For this review, take the finished solid that the model builds, in its own axes (mm). Round coordinates to 2 decimals unless told otherwise and drop trailing zeros. Write each loop counter-clockwise with the first axis right and the second up, starting at its lowest first coordinate (ties: lowest second). Pieces come first, ordered by that corner, then holes. Notation, with made-up numbers: M 36,78.25 L 92,78.25 A19 ccw 92,112.25 Z; hole C 47.25,-12 d1. An arc over 180 degrees is marked long. Use one line per item in the form item = value. Start each with the question number.
Item 1: Add section D-D (x = -52). State the section outline as (y, z) points, and give its area (3 significant figures).
Item 2: Add section A-A (z = -0.65). State the section outline as (x, y) points, and give its area (3 significant figures).
Item 3: Add section B-B (y = 0). State the section outline as (x, z) points.
Item 4: For line 1 (Y direction, x = -47, z = -0.8); line 2 (Y direction, x = -19, z = -0.4); line 3 (Y direction, x = -24, z = -0.65), list the stretches that pass through material, from the lowest coordinate up. Write a range as [from, to].
Item 5: Add section C-C (y = 40). State the section outline as (x, z) points, and give its area (4 significant figures).
Item 6: Draft analysis for pull direction X (two halves, no side actions). For faces 1 (the cylindrical face through (39.54, 40.11, -0.49)), 2 (the cylindrical face through (51.464, -48.985, -0.493)), 3 (the cylindrical face through (-21.66, 0.11, -0.49)), 4 (the flat face through (20, 4, 0)), state which applies: released by +X, released by -X, zero draft, split by the parting line, or undercut.
from build123d import *

# Parameters (mm, degrees)
SKETCH2_R          = 2.5
SKETCH2_R_2        = 2.25
BASE_FLANGE1_DEPTH = 1


# Sheet-metal steps are written as plain solids
with BuildPart() as part:
    # Sketch2 → Base-Flange1 (new body)
    with BuildSketch(Plane.XY):
        with BuildLine():
            Line((-62.163787728, 10), (13.698785388, 10))
            ThreePointArc((13.698785388, 10), (16.546759576, 10.890371912), (18.380431275, 13.244382792))
            Line((18.380431275, 13.244382792), (30.947144181, 46.755617208))
            ThreePointArc((30.947144181, 46.755617208), (32.78081588, 49.109628088), (35.628790069, 50))
            Line((35.628790069, 50), (48.443634474, 50))
            ThreePointArc((48.443634474, 50), (51.428287122, 49.011464641), (53.2327659, 46.436739428))
            Line((53.2327659, 46.436739428), (66.7327659, 1.436739428))
            ThreePointArc((66.7327659, 1.436739428), (66.943634474, 0), (66.7327659, -1.436739428))
            Line((66.7327659, -1.436739428), (53.2327659, -46.436739428))
            ThreePointArc((53.2327659, -46.436739428), (51.428287122, -49.011464641), (48.443634474, -50))
            Line((48.443634474, -50), (35.628790069, -50))
            ThreePointArc((35.628790069, -50), (32.78081588, -49.109628088), (30.947144181, -46.755617208))
            Line((30.947144181, -46.755617208), (18.380431275, -13.244382792))
            ThreePointArc((18.380431275, -13.244382792), (16.546759576, -10.890371912), (13.698785388, -10))
            Line((13.698785388, -10), (-62.163787728, -10))
            ThreePointArc((-62.163787728, -10), (-65.699321634, -8.535533906), (-67.163787728, -5))
            Line((-67.163787728, -5), (-67.163787728, 5))
            ThreePointArc((-67.163787728, 5), (-65.699321634, 8.535533906), (-62.163787728, 10))
        make_face()
        with Locations((-19.163787728, 0)):
            Circle(SKETCH2_R, mode=Mode.SUBTRACT)
        with Locations((42.036212272, 40)):
            Circle(SKETCH2_R, mode=Mode.SUBTRACT)
        with Locations((42.036212272, -40)):
            Circle(SKETCH2_R, mode=Mode.SUBTRACT)
        with Locations((-62.163787728, 0)):
            Circle(SKETCH2_R_2, mode=Mode.SUBTRACT)
        with Locations((-47.163787728, 0)):
            Circle(SKETCH2_R_2, mode=Mode.SUBTRACT)
        with Locations((8.836212272, 0)):
            Circle(SKETCH2_R_2, mode=Mode.SUBTRACT)
        with Locations((60.836212272, 0)):
            Circle(SKETCH2_R_2, mode=Mode.SUBTRACT)
    extrude(amount=-BASE_FLANGE1_DEPTH)


solid = part.part
Calculated:
q1.outline = M -10,-1 L 10,-1 L 10,0 L -10,0 Z
q1.area = 20.0 mm^2
q2.outline = M -67.16,-5 A5 ccw -62.16,-10 L 13.7,-10 A5 cw 18.38,-13.24 L 30.95,-46.76 A5 ccw 35.63,-50 L 48.44,-50 A5 ccw 53.23,-46.44 L 66.73,-1.44 A5 ccw 66.73,1.44 L 53.23,46.44 A5 ccw 48.44,50 L 35.63,50 A5 ccw 30.95,46.76 L 18.38,13.24 A5 cw 13.7,10 L -62.16,10 A5 ccw -67.16,5 Z; hole C -62.16,0 d4.5; hole C -47.16,0 d4.5; hole C -19.16,0 d5; hole C 8.84,0 d4.5; hole C 42.04,-40 d5; hole C 42.04,40 d5; hole C 60.84,0 d4.5
q2.area = 5,200 mm^2
q3.outline = M -67.16,-1 L -64.41,-1 L -64.41,0 L -67.16,0 Z; M -59.91,-1 L -49.41,-1 L -49.41,0 L -59.91,0 Z; M -44.91,-1 L -21.66,-1 L -21.66,0 L -44.91,0 Z; M -16.66,-1 L 6.59,-1 L 6.59,0 L -16.66,0 Z; M 11.09,-1 L 58.59,-1 L 58.59,0 L 11.09,0 Z; M 63.09,-1 L 66.94,-1 L 66.94,0 L 63.09,0 Z
q4.line_1 = [-10, -2.24], [2.24, 10]
q4.line_2 = [-10, -2.49], [2.49, 10]
q4.line_3 = [-10, 10]
q5.outline = M 28.41,-1 L 39.54,-1 L 39.54,0 L 28.41,0 Z; M 44.54,-1 L 55.16,-1 L 55.16,0 L 44.54,0 Z
q5.area = 21.75 mm^2
q6.face_1 = undercut
q6.face_2 = released by +X
q6.face_3 = undercut
q6.face_4 = zero draft
